Autodesk Inventor part; units mm, degrees
ref_plane "YZ Plane" through (0, 0, 0) normal (1, 0, 0) x (0, 1, 0)
ref_plane "XZ Plane" through (0, 0, 0) normal (0, 1, 0) x (-1, 0, 0)
ref_plane "XY Plane" through (0, 0, 0) normal (0, 0, 1) x (1, 0, 0)
sketch "Sketch1" plane through (0, 0, 0) normal (0, 0, 1) x (1, 0, 0)
  line L0 (2.3094, -4) -> (-2.3094, -4)
  line L1 (-2.3094, -4) -> (-4.6188, 0)
  line L2 (-4.6188, 0) -> (-2.3094, 4)
  line L3 (-2.3094, 4) -> (2.3094, 4)
  line L4 (2.3094, 4) -> (4.6188, 0)
  line L5 (4.6188, 0) -> (2.3094, -4)
  point P0 (0, 0)
  point P1 (0, 0)
  dimension "d0" = 8
extrude "Extrusion1" add sketch "Sketch1" along normal blind 10
sketch "Sketch2" plane through (0, 0, 10) normal (0, 0, 1) x (1, 0, 0)
  circle A0 centre (0, 0) radius 3.7
  dimension "d3" = 7.4
extrude "Extrusion2" add sketch "Sketch2" along normal blind 8
fillet "Fillet1" radius 0.4 1 edges at (-3.7, 0, 18)
properties part number "hex_shaft"
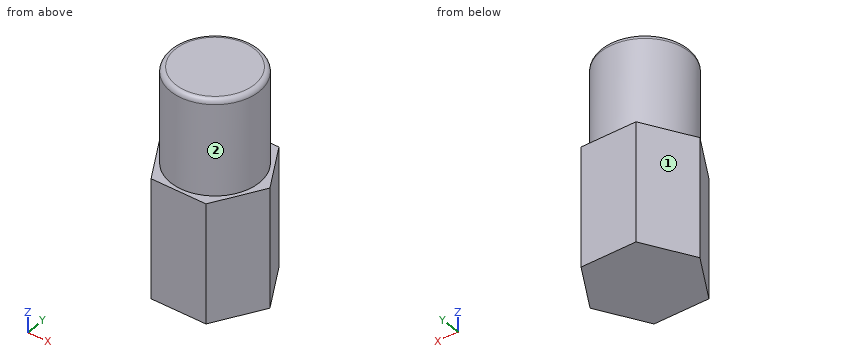
Can you work these out from the model? Positions are in its coordinate system, mm. Face numbers are marked on the shaded views. A direction names the side the tool comes from. Round coordinates to 2 decimals unless told otherwise and drop trailing zeros. Order: outer loops, then holes, each group sorted by start corner. A loop starts at its lowest first (then second) coordinate and runs counter-clockwise, first axis right, second up. Notation, with made-up numbers: (-22.5, -0.75) -> (18.5, -0.75) arc R13 ccw to (18.5, 10.25) -> close; hole circle Ø6 at (2.25, -8.75). An arc over 180 degrees is marked (long way). Write each question's results on one line, items separated by ' | '. Start each with the question number.
Item 1: Please list where these lines run through material, in increasing order: L1, parallel to X at y = -1.75, z = 1; L2, parallel to Y at x = -0.5, z = 13.5; L3, parallel to X at y = 3, z = 2.25.
Item 2: If we section it at A-A, the plane x = 0: Write out the boundary of the cut face in (y, z).
Item 3: If we section it at B-B, the plane z = 16: Write out the boundary of the cut face in (x, y).
Item 4: Which directions (+Z, -Z, +X, -X, +Y, -Y) give clear straight access to the entire face, cutting with the end or side of a thin tool? Please do the marked faces 1 and 2.
Item 5: If we section it at C-C, the plane z = 9: Write out the boundary of the cut face in (x, y).
Item 6: Will this pin go through, and if not, where does the flat tip stop? pin 1 (3 mm diameter, centred on y = 0, z = 15.5, fed in from -X).
Results:
1) L1: x = -3.61 to 3.61 | L2: y = -3.67 to 3.67 | L3: x = -2.89 to 2.89
2) outline: (-4, 0) -> (4, 0) -> (4, 10) -> (3.7, 10) -> (3.7, 17.6) arc R0.4 ccw to (3.3, 18) -> (-3.3, 18) arc R0.4 ccw to (-3.7, 17.6) -> (-3.7, 10) -> (-4, 10) -> close
3) outline: circle Ø7.4 at (0, 0)
4) face 1: +Z, -Z, -X, +Y | face 2: +Z
5) outline: (-4.62, 0) -> (-2.31, -4) -> (2.31, -4) -> (4.62, 0) -> (2.31, 4) -> (-2.31, 4) -> close
6) pin 1: stops at x = -3.7
